Design review of the part built by this model. Coordinates are the model's own, in mm. Round coordinates to 2 decimals unless told otherwise and drop trailing zeros. Order: outer loops, then holes, each group sorted by start corner. A loop starts at its lowest first (then second) coordinate and runs counter-clockwise, first axis right, second up. Notation, with made-up numbers: M -20,-9.5 L 8,-9.5 A23 cw 8,28.5 Z; hole C -13.5,0.5 d10. An arc over 180 degrees is marked long. Write item = value, one per line. Start each with the question number.
```python
from build123d import *

# Parameters (mm, degrees)
SKETCH1_W           = 33.274
SKETCH1_H           = 27.94
BOSS_EXTRUDE1_DEPTH = 2.54
SKETCH2_R           = 1.397
CUT_EXTRUDE1_DEPTH  = 2.54
FILLET1_R           = 3.81


with BuildPart() as part:
    # Sketch1 → Boss-Extrude1 (new body)
    with BuildSketch(Plane(origin=(0, 0, 0), x_dir=(1, 0, 0), z_dir=(0, 1, 0))):
        Rectangle(SKETCH1_W, SKETCH1_H)
    extrude(amount=BOSS_EXTRUDE1_DEPTH)

    # Sketch2 → Cut-Extrude1 (cut)
    with BuildSketch(Plane(origin=(0, 2.54, 0), x_dir=(1, 0, 0), z_dir=(0, 1, 0))):
        with Locations((12.7, -10.16)):
            Circle(SKETCH2_R)
        with Locations((-12.7, -10.16)):
            Circle(SKETCH2_R)
        with Locations((12.7, 10.16)):
            Circle(SKETCH2_R)
    extrude(amount=-CUT_EXTRUDE1_DEPTH, mode=Mode.SUBTRACT)

    # Fillet1
    fillet1_edges = [part.edges().sort_by_distance(p)[0] for p in [
        (16.637, 1.27, 13.97),
        (-16.637, 1.27, 13.97),
        (-16.637, 1.27, -13.97),
        (16.637, 1.27, -13.97),
    ]]
    fillet(fillet1_edges, radius=FILLET1_R)


solid = part.part
```
(1) Consider section B-B, the plane z = 10.75. Write out the cut boundary in (x, y), then the cut area to 3 significant figures.
(2) For line 1 along Z through (x, y) = (12.7, 0.65); line 2 along X through (y, z) = (1, 10.16); line 3 along X through (y, z) = (1.35, -10.16), list the stretches that pass through material, from the lowest coordinate up. Write a range as [from, to].
(3) Consider section D-D, the plane z = -9.75. Write out the cut boundary in (x, y), then the cut area to 3 significant figures.
(4) Insertion check: pin 1 (8 mm diameter, centred on x = -1.5, z = 4, fed in from -Y). The pin has a flat end and moves straight along its axis. Give the tip position at first contact, or say it passes through.
(5) Consider section C-C, the plane x = -12. Write out the cut boundary in (y, z), then the cut area to 3 significant figures.
(6) Consider section A-A, the plane y = 0.4. Write out the cut boundary in (x, z).
(7) Draft analysis for pull direction Z (two halves, no side actions). For faces 1 (the face through (0, 1, -13.97)), 2 (the face through (16.637, 1, 0)), 3 (the face through (12.397, 1.288, -8.796)), state which applies: pulls with the +Z half, pulls with the -Z half, needs draft (parallel to the pull), parting line crosses it, or undercut.
Completed:
q1.outline = M -16.59,0 L -13.97,0 L -13.97,2.54 L -16.59,2.54 Z; M -11.43,0 L 11.43,0 L 11.43,2.54 L -11.43,2.54 Z; M 13.97,0 L 16.59,0 L 16.59,2.54 L 13.97,2.54 Z
q1.area = 71.4 mm2
q2.line_1 = [-13.97, -11.56], [-8.76, 8.76], [11.56, 13.97]
q2.line_2 = [-16.64, -14.1], [-11.3, 11.3], [14.1, 16.64]
q2.line_3 = [-16.64, 11.3], [14.1, 16.64]
q3.outline = M -16.64,0 L 11.36,0 L 11.36,2.54 L -16.64,2.54 Z; M 14.04,0 L 16.64,0 L 16.64,2.54 L 14.04,2.54 Z
q3.area = 77.7 mm2
q4.pin_1 = 0
q5.outline = M 0,-13.97 L 2.54,-13.97 L 2.54,8.95 L 0,8.95 Z; M 0,11.37 L 2.54,11.37 L 2.54,13.97 L 0,13.97 Z
q5.area = 64.8 mm2
q6.outline = M -16.64,-10.16 A3.81 ccw -12.83,-13.97 L 12.83,-13.97 A3.81 ccw 16.64,-10.16 L 16.64,10.16 A3.81 ccw 12.83,13.97 L -12.83,13.97 A3.81 ccw -16.64,10.16 Z; hole C -12.7,10.16 d2.79; hole C 12.7,-10.16 d2.79; hole C 12.7,10.16 d2.79
q7.face_1 = pulls with the -Z half
q7.face_2 = needs draft
q7.face_3 = undercut
